from build123d import *

# Parameters (mm, degrees)
SKETCH006_W      = 5.741076
SKETCH006_H      = 2
EXTRUDE004_DEPTH = 1
CHAMFER_SIZE     = 1.6
EXTRUDE003_DEPTH = 7.5
SKETCH001_R      = 3.3
EXTRUDE001_DEPTH = 17
SKETCH002_R      = 5.75
EXTRUDE002_DEPTH = 2
SKETCH_R         = 1.7
EXTRUDE_DEPTH    = 1


with BuildPart() as chamfer_body:
    # Sketch006 → Extrude004 (new body, symmetric)
    with BuildSketch(Plane.YZ):
        with Locations((0, 3.5)):
            Rectangle(SKETCH006_W, SKETCH006_H)
    extrude(amount=EXTRUDE004_DEPTH, both=True)

    # Chamfer
    chamfer_edges = [chamfer_body.edges().sort_by_distance(p)[0] for p in [
        (1, 0, 4.5),
    ]]
    chamfer(chamfer_edges, length=CHAMFER_SIZE)


with BuildPart() as hole_e:
    # Sketch003 → Extrude003 (new body, symmetric)
    with BuildSketch(Plane.YZ):
        with BuildLine():
            Line((-1.975, 8.5), (-1.975, 4.487526))
            Line((-1.975, 4.487526), (-1.695672, 2.5))
            Line((-1.695672, 2.5), (0.001755, 2.5))
            Line((0.001755, 2.5), (1.699181, 2.5))
            Line((1.975, 4.462553), (1.699181, 2.5))
            Line((1.975, 8.5), (1.975, 4.462553))
            Line((1.975, 12.525), (1.975, 8.5))
            ThreePointArc((1.975, 12.525), (0, 14.5), (-1.975, 12.525))
            Line((-1.975, 12.525), (-1.975, 8.5))
        make_face()
    extrude(amount=EXTRUDE003_DEPTH, both=True)


with BuildPart() as slice2_e:
    # Sketch001 → Extrude001 (new body)
    with BuildSketch(Plane.XY.offset(1)):
        Circle(SKETCH001_R)
    extrude(amount=EXTRUDE001_DEPTH)


with BuildPart() as slice3_e:
    # Sketch002 → Extrude002 (new body)
    with BuildSketch(Plane.XY.offset(18)):
        Circle(SKETCH002_R)
    extrude(amount=EXTRUDE002_DEPTH)


with BuildPart() as everything:
    # Sketch → Extrude (new body)
    with BuildSketch(Plane.XY):
        Circle(SKETCH_R)
    extrude(amount=EXTRUDE_DEPTH)

    # Fusion: union slice2_e, slice3_e
    add(slice2_e.part)
    add(slice3_e.part)

    # Cut: cut hole_e
    add(hole_e.part, mode=Mode.SUBTRACT)

    # Fusion001: union Chamfer body
    add(chamfer_body.part)


solid = everything.part
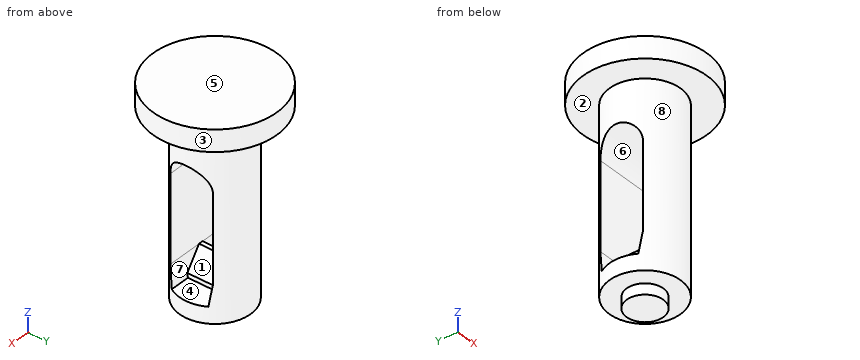
Can you work these out from the model? Positions are in its coordinate system, mm. Face numbers are marked on the shaded views. A direction names the side the tool comes from. Coordinates: 2 decimals unless noted, no trailing zeros. Order: outer loops, then holes, each group sorted by start corner. A loop starts at its lowest first (then second) coordinate and runs counter-clockwise, first axis right, second up. Notation, with made-up numbers: (-16.75, 14) -> (-10.75, 14) arc R4 ccw to (-10.75, 21) -> close; hole circle Ø6 at (-38.5, 72.5). An arc over 180 degrees is marked (long way). Use one line per item in the form item = value.
Q1. I need wall thicknesses on L1, parallel to Z at x = 3.5, y = -0.25; L2, parallel to Y at x = 0.25, z = 13.75; L3, parallel to X at y = -0.5, z = 2.75. Which ranges of each line are inside material? Lowest first, please.
From the geometry:
L1 = 18 to 20
L2 = -3.29 to -1.55, 1.55 to 3.29
L3 = -1 to 1
Q2. Imagine slicing it at C-C, the plane z = 5. List the corners of the cut face in (x, y) for me (3 decimals), then the cut area to 3 significant figures.
From the geometry:
outline = (-2.644, -1.975) arc R3.3 ccw to (2.644, -1.975) -> close; (-2.644, 1.975) -> (2.644, 1.975) arc R3.3 ccw to start
area = 9.79 mm²
Q3. Which directions (+Z, -Z, +X, -X, +Y, -Y) give clear straight access to the entire face, cutting with the end or side of a thin tool? Please do the marked faces 5, 6, 7 and 8.
From the geometry:
face_5 = +Z, +X, -X, +Y, -Y
face_6 = +X, -X
face_7 = +X
face_8 = -Z
Q4. Will these pins go through, and if not, where does the flat tip stop? P1, Ø2.5, axis at x = 0, z = 9.5, coming from the +Y side; P2, Ø6, axis at y = -2.5, z = 16.5, coming from the -X side; P3, Ø2, axis at y = -3, z = 12.5, coming from the +X side; P4, Ø1.6, axis at y = 0.5, z = 3, coming from the -X side.
From the geometry:
P1 = 3.3
P2 = -5.75
P3 = 2.62
P4 = -3.3
Q5. Imagine slicing it at B-B, the plane x = 0. List the corners of the cut face in (y, z) for me (3 decimals).
From the geometry:
outline = (-5.75, 18) -> (-3.3, 18) -> (-3.3, 1) -> (-1.7, 1) -> (-1.7, 0) -> (1.7, 0) -> (1.7, 1) -> (3.3, 1) -> (3.3, 18) -> (5.75, 18) -> (5.75, 20) -> (-5.75, 20) -> close; hole (-1.975, 4.488) -> (-1.892, 3.9) -> (1.896, 3.9) -> (1.975, 4.463) -> (1.975, 12.525) arc R1.975 ccw to (-1.975, 12.525) -> close
Q6. Imagine slicing it at D-D, the plane y = 2.25. List the corners of the cut face in (x, z) for me.
From the geometry:
outline = (-5.29, 18) -> (-2.41, 18) -> (-2.41, 1) -> (2.41, 1) -> (2.41, 18) -> (5.29, 18) -> (5.29, 20) -> (-5.29, 20) -> close
Q7. We'd pull the mould along Z, two halves only. Please class the marked faces 1, 2, 3 and 4: released by +Z, released by -Z, zero draft, split by the parting line, or undercut.
From the geometry:
face_1 = undercut
face_2 = released by -Z
face_3 = zero draft
face_4 = undercut
Q8. Imagine slicing it at A-A, the plane y = 0. List the corners of the cut face in (x, z) for me, then the cut area to 3 significant figures.
From the geometry:
outline = (-5.75, 18) -> (-3.3, 18) -> (-3.3, 14.5) -> (3.3, 14.5) -> (3.3, 18) -> (5.75, 18) -> (5.75, 20) -> (-5.75, 20) -> close; (-3.3, 1) -> (-1.7, 1) -> (-1.7, 0) -> (1.7, 0) -> (1.7, 1) -> (3.3, 1) -> (3.3, 2.5) -> (1, 2.5) -> (1, 2.9) -> (-0.6, 4.5) -> (-1, 4.5) -> (-1, 2.5) -> (-3.3, 2.5) -> close
area = 62.1 mm²
